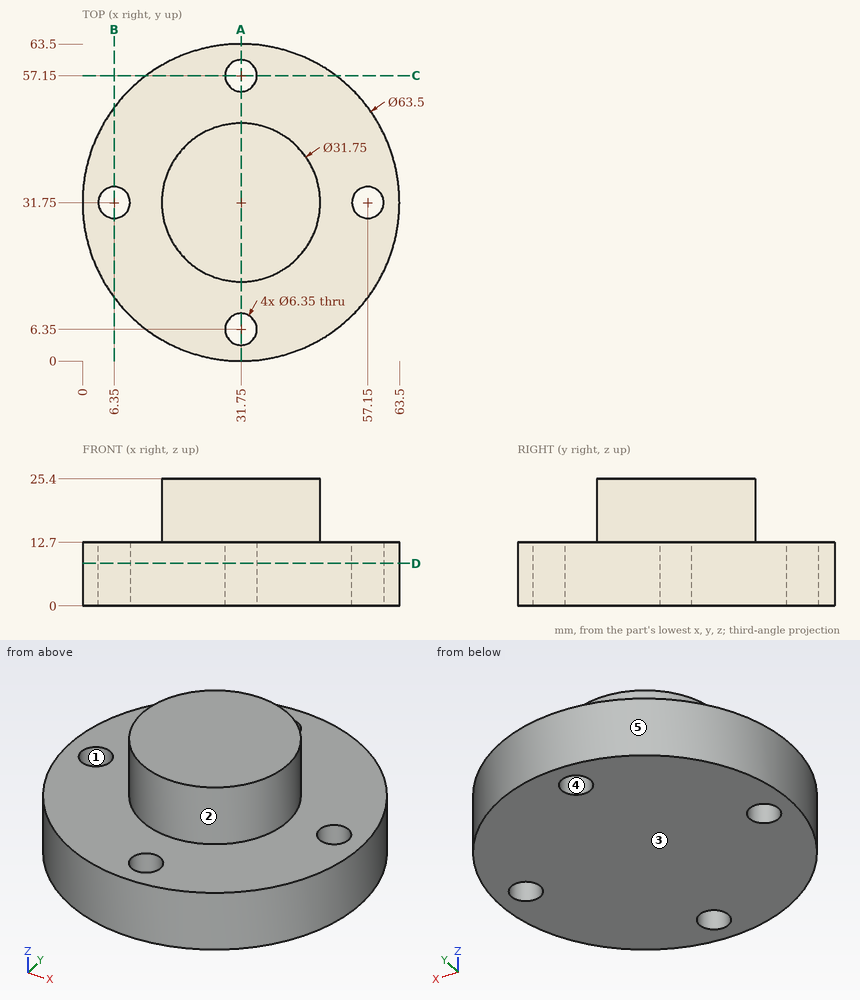
Verification items for this drawing (mm, ordinates from the low corner). A direction names the side the tool comes from. Coordinates: 2 decimals unless noted, no trailing zeros. Order: outer loops, then holes, each group sorted by start corner. A loop starts at its lowest first (then second) coordinate and runs counter-clockwise, first axis right, second up. Notation, with made-up numbers: M -7.5,-5 L 50.5,-5 A27 ccw 50.5,29 Z; hole C -4,-8.5 d10. An arc over 180 degrees is marked long. Use CSV: the item, a comma, the result in double quotes.
Item 1: Tool access check on the marked faces 1 and 2. Record the directions out of +Z, -Z, +X, -X, +Y, -Y that give a thin tool (end or side, any length) a straight path to the whole face; none if there is none.
Returned:
face 1,"+Z, -Z"
face 2,"+Z"
Item 2: Cross-section at B-B on x = 6.35. Record the cut outline in (y, z) (3 decimals).
Returned:
outline,"M 12.7,0 L 28.575,0 L 28.575,12.7 L 12.7,12.7 Z; M 34.925,0 L 50.8,0 L 50.8,12.7 L 34.925,12.7 Z"
Item 3: Gauge pin test, flat ends, axial feed: pin 1 Ø8 at (y, z) = (42.5, 11.5) entering from +X; pin 2 Ø6 at (x, z) = (32, 22) entering from +Y (3 decimals); pin 3 Ø3 at (x, y) = (39, 9) entering from -Z; pin 4 Ø1 at (x, y) = (45, 13.5) entering from +Z. Record the tip position at first contact, or that the pin passes through.
Returned:
pin 1,"stops at x = 62.77"
pin 2,"stops at y = 47.625"
pin 3,"stops at z = 0"
pin 4,"stops at z = 12.7"
Item 4: Thickness scan on line 1 along Y through (x, z) = (31.75, 3.5) (3 decimals); line 2 along Y through (x, z) = (29, 11.75); line 3 along Z through (x, y) = (42, 45.5). Record the ranges inside material, lowest first.
Returned:
line 1,"y = 0 to 3.175, 9.525 to 53.975, 60.325 to 63.5"
line 2,"y = 0.12 to 4.76, 7.94 to 55.56, 58.74 to 63.38"
line 3,"z = 0 to 12.7"
Item 5: Cross-section at A-A on x = 31.75. Record the cut outline in (y, z) (3 decimals).
Returned:
outline,"M 0,0 L 3.175,0 L 3.175,12.7 L 0,12.7 Z; M 9.525,0 L 53.975,0 L 53.975,12.7 L 47.625,12.7 L 47.625,25.4 L 15.875,25.4 L 15.875,12.7 L 9.525,12.7 Z; M 60.325,0 L 63.5,0 L 63.5,12.7 L 60.325,12.7 Z"
Item 6: Cross-section at D-D on z = 8.5. Record the cut outline in (x, y) (3 decimals), then the cut area to 3 significant figures.
Returned:
outline,"C 31.75,31.75 d63.5; hole C 6.35,31.75 d6.35; hole C 31.75,6.35 d6.35; hole C 31.75,57.15 d6.35; hole C 57.15,31.75 d6.35"
area,"3,040 mm2"
Item 7: Mould release check, pull along X, two halves, no side actions. Record for the marked faces 3, 4 and 5: pulls with the +X half, pulls with the -X half, needs draft (parallel to the pull), parting line crosses it, or undercut.
Returned:
face 3,"needs draft"
face 4,"undercut"
face 5,"parting line crosses it"
